Could you check a few things on this model? Use its own coordinates, in mm. A direction names the side the tool comes from. Give positions to 0.01 mm unless a question says otherwise; leave off trailing zeros. Write each loop counter-clockwise with the first axis right and the second up, starting at its lowest first coordinate (ties: lowest second). Pieces come first, ordered by that corner, then holes. Notation, with made-up numbers: (30, -0.5) - (52, -0.5) arc R15 cw to (52, 24.5) - close; hole circle Ø6 at (20, 36.25). An arc over 180 degrees is marked (long way). Use one line per item in the form item = value.
```python
from build123d import *

# Parameters (mm, degrees)
SKETCH_6_R          = 7.5
EXTRUDE_1_DEPTH     = 3
SKETCH_7_R          = 4.5
SKETCH_7_R_2        = 3.15
EXTRUDE_2_DEPTH     = 10
FILLET_1_R          = 3
SKETCH_9_R          = 1.65
CUT_EXTRUDE_1_DEPTH = 3
FILLET_2_R          = 1
SKETCH_10_R         = 1.35
CUT_EXTRUDE_2_DEPTH = 37.90351326


with BuildPart() as part:
    # 草图6 → 凸台-拉伸1 (new body)
    with BuildSketch(Plane.XY):
        with Locations((18.143108258, 29.936835998)):
            Circle(SKETCH_6_R)
    extrude(amount=EXTRUDE_1_DEPTH)

    # 草图7 → 凸台-拉伸2 (add)
    with BuildSketch(Plane.XY.offset(3)):
        with Locations((18.143108258, 29.936835998)):
            Circle(SKETCH_7_R)
        with Locations((18.143108258, 29.936835998)):
            Circle(SKETCH_7_R_2, mode=Mode.SUBTRACT)
    extrude(amount=EXTRUDE_2_DEPTH)

    # 圆角1
    fillet_1_edges = [part.edges().sort_by_distance(p)[0] for p in [
        (13.643108258, 29.936835998, 3),
    ]]
    fillet(fillet_1_edges, radius=FILLET_1_R - 0.0001)  # a hair under: the kernel refuses the full size

    # 草图9 → 切除-拉伸1 (cut)
    with BuildSketch(Plane.XY.offset(3)):
        with Locations((18.143108258, 29.936835998)):
            Circle(SKETCH_9_R)
    extrude(amount=-CUT_EXTRUDE_1_DEPTH, mode=Mode.SUBTRACT)

    # 圆角2
    fillet_2_edges = [part.edges().sort_by_distance(p)[0] for p in [
        (10.643108258, 29.936835998, 3),
        (13.643108258, 29.936835998, 13),
    ]]
    fillet(fillet_2_edges, radius=FILLET_2_R)

    # 草图10 → 切除-拉伸2 (cut, through all)
    with BuildSketch(Plane(origin=(18.921476442, 3.905687751, 0), x_dir=(0, 0, 1), z_dir=(-0.9793537694565077, -0.20215388754938593, 0))):
        with Locations(Location((9, 25.651053313, 0), (0, 0, 270))):
            Circle(SKETCH_10_R)
    extrude(amount=-CUT_EXTRUDE_2_DEPTH, mode=Mode.SUBTRACT)


solid = part.part
```
1. For pin 1 (1.5 mm diameter, centred on x = 23.5, z = 3.5, fed in from -Y); pin 2 (2 mm diameter, centred on y = 32.5, z = 9, fed in from -X); pin 3 (5 mm diameter, centred on x = 18.14, y = 29.94, fed in from +Z), each with a flat end and sliding along its axis, tell me the tip position at first contact or that it passes through.
Response values:
pin_1 = 24.75
pin_2 = 13.92
pin_3 = 3
2. If I drill on line 1 (Y direction, x = 20.75, z = 7.5); line 2 (X direction, y = 27.75, z = 3.5); line 3 (Y direction, x = 17, z = 11.75), over which ranges is the centre line in solid material (lowest first)? Write a range as from..to.
Response values:
line_1 = 26.27..28.17, 31.71..33.6
line_2 = 12.73..15.88, 20.41..23.56
line_3 = 25.58..27, 32.87..34.29
3. If we mould it in two halves opening along Y, with no side actions, what happens to faces 1 (the face through (16, 30, 0)), 2 (the face through (17.168, 25.544, 8.958)), 3 (the face through (14.79, 27.93, 9.41))? For each: pulls with the +Y half, pulls with the -Y half, needs draft (parallel to the pull), parting line crosses it, or undercut.
Response values:
face_1 = needs draft
face_2 = parting line crosses it
face_3 = undercut
4. Which directions (+Z, -Z, +X, -X, +Y, -Y) give clear straight access to the entire face, cutting with the end or side of a thin tool? Please do faces 4 (the face through (19.5, 28.6, 3)), 5 (the face through (17.167, 37.373, 1.049)).
Response values:
face_4 = +Z
face_5 = +Z, -Z
5. Imagine slicing it at D-D, the plane z = 1.25. List the corners of the cut face in (x, y) for me.
Response values:
outline = circle Ø15 at (18.14, 29.94); hole circle Ø3.3 at (18.14, 29.94)
6. Imagine slicing it at C-C, the plane z = 7. List the corners of the cut face in (x, y) for me.
Response values:
outline = circle Ø9 at (18.14, 29.94); hole circle Ø6.3 at (18.14, 29.94)
7. Imagine slicing it at B-B, the plane y = 31.25. State how many separate pieces and enclosed holes the cut face has, and give its area (3 significant figures).
Response values:
separate_pieces = 3
enclosed_holes = 0
area = 66.9 mm²
8. Imagine slicing it at A-A, the plane z = 9.25. List the corners of the cut face in (x, y) for me, and give its area (3 significant figures).
Response values:
outline = (13.66, 30.37) - (15.08, 30.66) arc R3.15 cw to (20.67, 31.81) - (22.09, 32.11) arc R4.5 ccw to start; (14.2, 27.77) arc R4.5 ccw to (22.62, 29.51) - (21.21, 29.22) arc R3.15 cw to (15.61, 28.06) - close
area = 25.1 mm²
